Read the model definition and answer for the solid it produces. Units are mm, in the model's axes. A direction names the side the tool comes from. Give positions to 0.01 mm unless a question says otherwise; leave off trailing zeros. Order: outer loops, then holes, each group sorted by start corner. A loop starts at its lowest first (then second) coordinate and runs counter-clockwise, first axis right, second up. Notation, with made-up numbers: M 7.5,18.5 L 50.5,18.5 A27 cw 50.5,39.5 Z; hole C 59,-13 d2. An arc over 180 degrees is marked long. One line per item, written item: value.
from build123d import *

# Parameters (mm, degrees)
SKETCH1_W = 6
SKETCH1_H = 5
SKETCH3_W = 0.5
SKETCH3_H = 3


with BuildPart() as part:
    # Sketch1 → Revolve1 (revolve)
    with BuildSketch(Plane(origin=(0, 0, 0), x_dir=(0, 0, -1), z_dir=(1, 0, 0)), mode=Mode.PRIVATE) as revolve1_sk:
        with Locations((0, 22.5)):
            Rectangle(SKETCH1_W, SKETCH1_H)
    revolve(revolve1_sk.sketch.rotate(Axis((0, 0, 0), (0, 0, -1)), 90), axis=Axis((0, 0, 0), (0, 0, -1)))

    # Sketch3 → Cut-Revolve2 (revolve, cut)
    with BuildSketch(Plane(origin=(0, 0, 0), x_dir=(0, 0, -1), z_dir=(1, 0, 0)), mode=Mode.PRIVATE) as cut_revolve2_sk:
        with Locations((2.75, 22.5)):
            Rectangle(SKETCH3_W, SKETCH3_H)
        with Locations((-2.75, 22.5)):
            Rectangle(SKETCH3_W, SKETCH3_H)
    revolve(cut_revolve2_sk.sketch.rotate(Axis((0, 0, 0), (0, 0, -1)), 90), axis=Axis((0, 0, 0), (0, 0, -1)), mode=Mode.SUBTRACT)


solid = part.part
1) Each of these flat-tipped pins is pushed along its axis until it touches: pin 1 Ø3 at (x, y) = (4, -18) entering from -Z; pin 2 Ø1.5 at (y, z) = (-1.5, -0.5) entering from +X; pin 3 Ø2 at (y, z) = (11, 2) entering from +X; pin 4 Ø1.5 at (x, z) = (-11, 1.5) entering from +Y. Where does it stop, or does it pass through?
Reported:
pin 1: passes through
pin 2: stops at x = 24.99
pin 3: stops at x = 22.91
pin 4: stops at y = 22.8
2) Find section C-C, the plane z = 1.45. Write down the section's boundary in (x, y).
Reported:
outline: C 0,0 d50; hole C 0,0 d40
3) Find section A-A, the plane y = 0. Write down the section's boundary in (x, z).
Reported:
outline: M -25,-3 L -24,-3 L -24,-2.5 L -21,-2.5 L -21,-3 L -20,-3 L -20,3 L -21,3 L -21,2.5 L -24,2.5 L -24,3 L -25,3 Z; M 20,-3 L 21,-3 L 21,-2.5 L 24,-2.5 L 24,-3 L 25,-3 L 25,3 L 24,3 L 24,2.5 L 21,2.5 L 21,3 L 20,3 Z
4) Which of the six approach directions +Z, -Z, +X, -X, +Y, -Y give full straight-line access (tool end or side, diameter ignored) to faces 4 (the face through (-19, 8, 3)), 5 (the face through (22.89, -7.21, 2.75)), 6 (the face through (20.03, -6.31, -2.75))?
Reported:
face 4: +Z, +X, -X, +Y, -Y
face 5: +Z
face 6: -Z
5) Find section D-D, the plane y = 22. Write down the section's boundary in (x, z), plus the area to 3 significant figures.
Reported:
outline: M -11.87,-3 L -9.59,-3 L -9.59,-2.5 L 9.59,-2.5 L 9.59,-3 L 11.87,-3 L 11.87,3 L 9.59,3 L 9.59,2.5 L -9.59,2.5 L -9.59,3 L -11.87,3 Z
area: 123 mm^2
6) Consider probe 1 along Y at (x, z) = (0, 2.85); probe 2 along Y at (x, z) = (0, 0); probe 3 along X at (y, z) = (0.5, -2.15) (3 decimals). Determine where each line is inside the solid, lowest interval first.
Reported:
probe 1: y = -25 to -24, -21 to -20, 20 to 21, 24 to 25
probe 2: y = -25 to -20, 20 to 25
probe 3: x = -24.995 to -19.994, 19.994 to 24.995
7) Determine the mould class of faces 1 (the face through (23.846, -7.509, -0.042)), 2 (the face through (0.1, 21.2, 2.5)), 3 (the face through (-19, 8, -3)) for opening direction X: +X half, -X half, draft (parallel to the pull), parting line (faces both ways), or undercut.
Reported:
face 1: parting line
face 2: undercut
face 3: draft
